For this review, take the finished solid that the model builds, in its own axes (mm). A direction names the side the tool comes from. Give positions to 0.01 mm unless a question says otherwise; leave off trailing zeros. Write each loop counter-clockwise with the first axis right and the second up, starting at its lowest first coordinate (ties: lowest second). Pieces come first, ordered by that corner, then holes.
Q1. For line 1 (X direction, y = -11.75, z = 11); line 2 (Y direction, x = 25, z = 9); line 3 (Z direction, x = 14, y = -7.5), list the stretches that pass through material, from the lowest coordinate up.
Q2. Mouldability with a two-part tool opening along X and no side actions: class faces 1 (the flat face through (0, -13, 17)), 2 (the cylindrical face through (50.316, -15.132, 6.439)), 3 (the flat face through (21.5, -18.2, 0)), 4 (the cylindrical face through (56.322, -12.432, 6.439)) as released by +X, released by -X, zero draft, split by the parting line, or undercut.
Q3. We need section A-A (y = -12.7). Write out the cut boundary in (x, z), then the cut area to 3 significant figures.
Q4. We need section C-C (z = 35.5). Write out the cut boundary in (x, y), then the cut area to 3 significant figures.
Q5. We need section D-D (x = 11). Write out the cut boundary in (y, z).
Q6. We need section B-B (x = 50). Write out the cut boundary in (y, z), then the cut area to 3 significant figures.
Q7. Machinability: for faces 5 (the flat face through (6, -19.05, 37)), 6 (the flat face through (35, -13, 12.7)), 7 (the cylindrical face through (20.36, -16.56, 6.44)), which of the approach directions +Z, -Z, +X, -X, +Y, -Y give a long, thin tool a straight path to every point of the face, cutting with its end or side? Answer none if there is none.
Q8. Insertion check: P1, Ø7.5, axis at y = -7.5, z = 31, coming from the +X side; P2, Ø5, axis at x = 5, z = 39, coming from the +Y side; P3, Ø8, axis at x = 6, z = 38, coming from the -Y side. Each pin has a flat end and moves straight along its axis. Give the tip position at first contact, or say it passes through.
```python
from build123d import *

# Parameters (mm, degrees)
F1_DEPTH = 25.4
F3_DEPTH = 25.4
F4_R     = 6.35
F5_DEPTH = 25.4


with BuildPart() as f1:
    # F0 (on Front) → F1 (new body)
    with BuildSketch(Plane.XZ):
        Polygon((0, 44.45), (0, 0), (57.15, 0), (57.15, 12.7), (12.7, 12.7), (12.7, 44.45), align=None)
    extrude(amount=F1_DEPTH)

    # F2 (on face) → F3 (cut)
    with BuildSketch(Plane.YZ.offset(12.7)):
        with BuildLine():
            ThreePointArc((-25.4, 32.1648232639), (-23.4956230285, 38.0400795664), (-19.05, 42.3274708663))
            Line((-19.05, 42.3274708663), (-19.05, 44.45))
            Line((-19.05, 44.45), (-25.4, 44.45))
            Line((-25.4, 44.45), (-25.4, 32.1648232639))
        make_face()
        with BuildLine():
            ThreePointArc((-19.05, 32.1648232639), (-12.7, 38.5148232639), (-6.35, 32.1648232639))
            Line((-6.35, 32.1648232639), (-6.35, 42.3274708663))
            ThreePointArc((-6.35, 42.3274708663), (-12.7, 44.0243544316), (-19.05, 42.3274708663))
            Line((-19.05, 42.3274708663), (-19.05, 32.1648232639))
        make_face()
        with BuildLine():
            ThreePointArc((-19.05, 42.3274708663), (-12.7, 44.0243544316), (-6.35, 42.3274708663))
            Line((-6.35, 42.3274708663), (-6.35, 44.45))
            Line((-6.35, 44.45), (-19.05, 44.45))
            Line((-19.05, 44.45), (-19.05, 42.3274708663))
        make_face()
        with BuildLine():
            ThreePointArc((-19.05, 32.1648232639), (-12.7, 25.8148232639), (-6.35, 32.1648232639))
            ThreePointArc((-6.35, 32.1648232639), (-12.7, 38.5148232639), (-19.05, 32.1648232639))
        make_face()
        with BuildLine():
            Line((-6.35, 44.45), (-6.35, 42.3274708663))
            ThreePointArc((-6.35, 42.3274708663), (-1.9043769715, 38.0400795664), (0, 32.1648232639))
            Line((0, 32.1648232639), (0, 44.45))
            Line((0, 44.45), (-6.35, 44.45))
        make_face()
    extrude(amount=-F3_DEPTH, mode=Mode.SUBTRACT)

    # F4 (on face) → F5 (cut)
    with BuildSketch(Plane.XY.offset(12.7)):
        with Locations((25.4, -12.7)):
            Circle(F4_R)
        with Locations((44.45, -12.7)):
            Circle(F4_R)
        with BuildLine():
            ThreePointArc((44.45, 0), (56.3249263826, -12.7), (44.45, -25.4))
            Line((44.45, -25.4), (57.15, -25.4))
            Line((57.15, -25.4), (57.15, 0))
            Line((57.15, 0), (44.45, 0))
        make_face()
    extrude(amount=-F5_DEPTH, mode=Mode.SUBTRACT)


solid = f1.part
```
Computed:
1. line 1: x = 0 to 19.12, 31.68 to 38.17, 50.73 to 56.29
1. line 2: y = -25.4 to -19.04, -6.36 to 0
1. line 3: z = 0 to 12.7
2. face 1: released by -X
2. face 2: undercut
2. face 3: zero draft
2. face 4: released by +X
3. outline: (0, 0) - (19.05, 0) - (19.05, 12.7) - (12.7, 12.7) - (12.7, 25.81) - (0, 25.81) - close; (31.75, 0) - (38.1, 0) - (38.1, 12.7) - (31.75, 12.7) - close; (50.8, 0) - (56.32, 0) - (56.32, 12.7) - (50.8, 12.7) - close
3. area: 559 mm2
4. outline: (0, -24.72) - (12.7, -24.72) - (12.7, -19.05) - (0, -19.05) - close; (0, -6.35) - (12.7, -6.35) - (12.7, -0.68) - (0, -0.68) - close
4. area: 144 mm2
5. outline: (-25.4, 0) - (0, 0) - (0, 32.16) arc R12.73 ccw to (-6.35, 42.33) - (-6.35, 32.16) arc R6.35 cw to (-19.05, 32.16) - (-19.05, 42.33) arc R12.73 ccw to (-25.4, 32.16) - close
6. outline: (-23.7, 0) - (-15.79, 0) - (-15.79, 12.7) - (-23.7, 12.7) - close; (-9.61, 0) - (-1.7, 0) - (-1.7, 12.7) - (-9.61, 12.7) - close
6. area: 201 mm2
7. face 5: +Z, +X, -X
7. face 6: +Z, +X, +Y, -Y
7. face 7: +Z, -Z
8. P1: stops at x = 12.7
8. P2: stops at y = -1.08
8. P3: stops at y = -25.14
